from build123d import *

# Parameters (mm, degrees)
BOSS_EXTRUDE1_DEPTH = 5.9944
SKETCH2_R           = 5.08
CUT_EXTRUDE1_DEPTH  = 372.756512027
CUT_EXTRUDE2_DEPTH  = 1.27
FILLET1_R           = 6.35


with BuildPart() as part:
    # Sketch1 → Boss-Extrude1 (new body)
    with BuildSketch(Plane(origin=(0, 0, 0), x_dir=(1, 0, 0), z_dir=(0, 1, 0))):
        Polygon((-66.675, 0), (66.675, 0), (108.238677943, -355.6), (-108.238677943, -355.6), align=None)
    extrude(amount=BOSS_EXTRUDE1_DEPTH)

    # Sketch2 → Cut-Extrude1 (cut, through all)
    with BuildSketch(Plane(origin=(0, 5.9944, 0), x_dir=(1, 0, 0), z_dir=(0, 1, 0))):
        with Locations(Location((0, -101.6, 0), (0, 0, 270))):
            Circle(SKETCH2_R)
    extrude(amount=-CUT_EXTRUDE1_DEPTH, mode=Mode.SUBTRACT)

    # Sketch3 → Cut-Extrude2 (cut)
    with BuildSketch(Plane(origin=(0, 5.9944, 0), x_dir=(1, 0, 0), z_dir=(0, 1, 0))):
        with BuildLine():
            Line((-0.64745098, -125.73), (-7.022352941, -125.73))
            add(Edge.make_bspline(
                [(-7.022352941, -125.73), (-6.995700037, -125.56647139), (-6.94264637, -125.240961184), (-6.822439521, -124.833851847), (-6.660985096, -124.502541973), (-6.475064564, -124.222842773), (-6.235482524, -123.909374898), (-5.933210944, -123.565961589), (-5.569119359, -123.193461978), (-5.137584514, -122.795086731), (-4.639123135, -122.372704423), (-4.278935295, -122.089977316), (-4.090147059, -121.941789216)],
                knots=[0, 0, 0, 0, 1.00794059, 2.006345856, 2.568221262, 3.244176762, 4.045978883, 4.967707078, 6.025786227, 7.214078669, 8.539791974, 10, 10, 10, 10], degree=3))
            add(Edge.make_bspline(
                [(-4.090147059, -121.941789216), (-3.959237505, -121.839291022), (-3.712095896, -121.645786669), (-3.367780634, -121.370812364), (-3.073520037, -121.12638684), (-2.749807849, -120.849934026), (-2.401956914, -120.521669006), (-2.050459284, -120.119964738), (-1.769921232, -119.720001197), (-1.574792785, -119.317093709), (-1.462696622, -118.90576348), (-1.450487068, -118.627391436), (-1.444313725, -118.486642157)],
                knots=[0, 0, 0, 0, 1.105083233, 2.086265203, 2.928643677, 3.647492745, 4.915719202, 6.103603942, 7.190110835, 8.152548768, 9.065899631, 10, 10, 10, 10], degree=3))
            add(Edge.make_bspline(
                [(-1.444313725, -118.486642157), (-1.447965678, -118.383696155), (-1.455062496, -118.183641793), (-1.508208178, -117.89411156), (-1.598896834, -117.626810225), (-1.725875028, -117.381877206), (-1.879897972, -117.157206868), (-2.067602091, -116.959226462), (-2.280144186, -116.783379567), (-2.521172126, -116.634524628), (-2.784585903, -116.511539466), (-3.072628503, -116.429562416), (-3.379272721, -116.373277743), (-3.591834853, -116.369040126), (-3.701053922, -116.366862745)],
                knots=[0, 0, 0, 0, 1.066440105, 2.072406788, 3.038089023, 3.980626898, 4.923164774, 5.851240192, 6.79842777, 7.774055624, 8.779619978, 9.800248095, 10.869719403, 12, 12, 12, 12], degree=3))
            add(Edge.make_bspline(
                [(-3.701053922, -116.366862745), (-3.856272912, -116.372784339), (-4.153856816, -116.384137145), (-4.575842478, -116.488503349), (-4.94872481, -116.662202163), (-5.273158686, -116.90555858), (-5.541086806, -117.223699711), (-5.760536331, -117.605911882), (-5.924737114, -118.058408876), (-5.991270058, -118.385922919), (-6.02627451, -118.558235294)],
                knots=[0, 0, 0, 0, 1.052503955, 2.0178474, 2.928593632, 3.828899676, 4.748107049, 5.732867451, 6.807211463, 8, 8, 8, 8], degree=3))
            Line((-6.02627451, -118.558235294), (-6.823137255, -118.43372549))
            add(Edge.make_bspline(
                [(-6.823137255, -118.43372549), (-6.80933515, -118.324490516), (-6.782336166, -118.110810556), (-6.71294302, -117.80167694), (-6.623223382, -117.510865089), (-6.510230906, -117.238067127), (-6.37723078, -116.983643092), (-6.222961391, -116.746154212), (-6.045126303, -116.528535029), (-5.846128896, -116.329076963), (-5.627309849, -116.151961167), (-5.393797446, -115.994859502), (-5.142464654, -115.86447923), (-4.877381927, -115.754431463), (-4.595667611, -115.670607699), (-4.298686261, -115.611680986), (-3.986147006, -115.577611658), (-3.772730074, -115.57257374), (-3.66370098, -115.57)],
                knots=[0, 0, 0, 0, 1.11558569, 2.182252598, 3.206865404, 4.197163727, 5.171016007, 6.113287932, 7.062752653, 8.014719109, 8.96418383, 9.912249364, 10.862587531, 11.829428462, 12.817713982, 13.836697005, 14.894825442, 16, 16, 16, 16], degree=3))
            add(Edge.make_bspline(
                [(-3.66370098, -115.57), (-3.556720592, -115.572319789), (-3.346239788, -115.576883907), (-3.037889894, -115.614942211), (-2.744018161, -115.6768103), (-2.465296832, -115.763662981), (-2.202890774, -115.877884746), (-1.951202346, -116.010088278), (-1.717482433, -116.17490368), (-1.497639325, -116.359297976), (-1.299748734, -116.564753592), (-1.122645846, -116.782681404), (-0.976555662, -117.018893798), (-0.853169483, -117.266964655), (-0.764695454, -117.53292748), (-0.694872253, -117.809240088), (-0.653577585, -118.101497133), (-0.649522593, -118.30078564), (-0.64745098, -118.402598039)],
                knots=[0, 0, 0, 0, 1.106681904, 2.177364475, 3.209175827, 4.210887483, 5.192078542, 6.167200624, 7.147039734, 8.145062256, 9.132109826, 10.094560107, 11.044836899, 12.000375742, 12.954465884, 13.938765234, 14.946957558, 16, 16, 16, 16], degree=3))
            add(Edge.make_bspline(
                [(-0.64745098, -118.402598039), (-0.651019305, -118.525228757), (-0.6580732, -118.767646194), (-0.715129167, -119.12624646), (-0.813824447, -119.47254261), (-0.943374808, -119.810657932), (-1.113892336, -120.134164725), (-1.314350095, -120.448008584), (-1.547654564, -120.749083332), (-1.770342076, -120.99003171), (-1.97351953, -121.182307301), (-2.148031694, -121.345116208), (-2.346754424, -121.522181935), (-2.570668292, -121.711175794), (-2.818646639, -121.913074715), (-3.084581883, -122.135434202), (-3.377659732, -122.368392422), (-3.582554579, -122.526226013), (-3.688602941, -122.607916667)],
                knots=[0, 0, 0, 0, 1.088993338, 2.152731221, 3.214950677, 4.282992305, 5.363056107, 6.45734114, 7.587448717, 8.741912054, 9.367708333, 10.072059012, 10.861970471, 11.731730561, 12.674646287, 13.702521352, 14.810883478, 16, 16, 16, 16], degree=3))
            add(Edge.make_bspline(
                [(-3.688602941, -122.607916667), (-3.814880187, -122.707673071), (-4.061272368, -122.90231778), (-4.409564614, -123.201952264), (-4.73097902, -123.495186281), (-5.017964452, -123.789920338), (-5.277411759, -124.07905832), (-5.50700849, -124.36473001), (-5.710619134, -124.64507084), (-5.822395863, -124.838757211), (-5.876862745, -124.933137255)],
                knots=[0, 0, 0, 0, 1.201760701, 2.344875646, 3.430713183, 4.449969728, 5.415927222, 6.330865599, 7.186659457, 8, 8, 8, 8], degree=3))
            Line((-5.876862745, -124.933137255), (-0.64745098, -124.933137255))
            Line((-0.64745098, -124.933137255), (-0.64745098, -125.73))
        make_face()
        with BuildLine():
            add(Edge.make_bspline(
                [(7.121960784, -116.348186275), (6.966339865, -116.529937257), (6.658951614, -116.888938584), (6.220934138, -117.43618394), (5.820990618, -117.99084912), (5.449181724, -118.546249507), (5.106128688, -119.103037308), (4.794532343, -119.662337897), (4.516462749, -120.225992354), (4.26698415, -120.792977059), (4.044548147, -121.3683878), (3.850270964, -121.955372575), (3.67057882, -122.552241729), (3.519790538, -123.16358515), (3.387268651, -123.786079212), (3.284032091, -124.423321677), (3.193868357, -125.071600422), (3.156448534, -125.509818618), (3.137647059, -125.73)],
                knots=[0, 0, 0, 0, 1.105388324, 2.183404297, 3.237157451, 4.263515625, 5.270618974, 6.257661546, 7.220201142, 8.173180298, 9.11857031, 10.06900231, 11.029056015, 11.99749775, 12.977109533, 13.9684726, 14.979265319, 16, 16, 16, 16], degree=3))
            Line((3.137647059, -125.73), (2.340784314, -125.73))
            add(Edge.make_bspline(
                [(2.340784314, -125.73), (2.370678975, -125.349642584), (2.429735016, -124.598257492), (2.61102689, -123.492894729), (2.858878127, -122.422284677), (3.182435664, -121.380929429), (3.581330157, -120.3591781), (3.949835575, -119.60787323), (4.230188707, -119.095806913), (4.404577952, -118.809755188), (4.594967573, -118.495142394), (4.815641098, -118.158570547), (5.057471949, -117.794755527), (5.324466786, -117.406124805), (5.619249624, -116.995425039), (5.821900516, -116.712397552), (5.926666667, -116.566078431)],
                knots=[0, 0, 0, 0, 1.601249526, 3.163222193, 4.697516546, 6.211791823, 7.737472103, 9.298034817, 9.721151344, 10.188082837, 10.704348124, 11.265001787, 11.877561367, 12.538519795, 13.244446179, 14, 14, 14, 14], degree=3))
            Line((5.926666667, -116.566078431), (0.94627451, -116.566078431))
            Line((0.94627451, -116.566078431), (0.94627451, -115.769215686))
            Line((0.94627451, -115.769215686), (7.121960784, -115.769215686))
            Line((7.121960784, -115.769215686), (7.121960784, -116.348186275))
        make_face()
    extrude(amount=-CUT_EXTRUDE2_DEPTH, mode=Mode.SUBTRACT)

    # Fillet1
    fillet1_edges = [part.edges().sort_by_distance(p)[0] for p in [
        (108.238677943, 2.9972, 355.6),
        (-108.238677943, 2.9972, 355.6),
        (-66.675, 2.9972, 0),
        (66.675, 2.9972, 0),
    ]]
    fillet(fillet1_edges, radius=FILLET1_R)


solid = part.part
Check sheet for the modelled part. Datum: model origin and axes. Units: mm. Round coordinates to 2 decimals unless told otherwise and drop trailing zeros. Loops run counter-clockwise (first coordinate to the right, second up) from the corner with the lowest first, then second, coordinate; pieces in that order, holes last. Notation, with made-up numbers: (-39.75, -26) -> (-2.75, -26) arc R20 cw to (-2.75, -3) -> close; hole circle Ø9 at (-17, 64.25). An arc over 180 degrees is marked (long way). Put each result on its own line as item: value. Start each with the question number.
1. Section check D-D (z = 247.5). Enter the section's corners in (x, y), plus the area to 3 significant figures.
2. Scan lines: probe 1 along X at (y, z) = (3.2, 101.6); probe 2 along X at (y, z) = (3.15, 136); probe 3 along X at (y, z) = (3.3, 313). Record each from-to range of solid material in increasing order.
3. Section check B-B (y = 1.55). Enter the section's corners in (x, z).
4. Section check C-C (x = -91.5). Enter the section's corners in (y, z), plus the area to 3 significant figures.
5. Draft check along Z on faces 1 (the face through (-87.65, 2.96, 179.46)), 2 (the face through (2, 0, 175)), 3 (the face through (1.526, 3.039, 106.445)). Enter one of: +Z half, -Z half, draft (parallel to the pull), parting line (faces both ways), or undercut.
6. Section check A-A (z = 101.6). Enter the section's corners in (x, y).
7. Gauge pin test, flat ends, axial feed: pin 1 (0.6 mm diameter, centred on y = 5.5, z = 125, fed in from -X); pin 2 (3 mm diameter, centred on y = 3, z = 193.5, fed in from -X); pin 3 (3 mm diameter, centred on y = 1, z = 169, fed in from +X). Record the tip position at first contact, or that the pin passes through.
Findings:
1. outline: (-95.6, 0) -> (95.6, 0) -> (95.6, 5.99) -> (-95.6, 5.99) -> close
1. area: 1,150 mm^2
2. probe 1: x = -78.55 to -5.08, 5.08 to 78.55
2. probe 2: x = -82.57 to 82.57
2. probe 3: x = -103.26 to 103.26
3. outline: (-107.41, 348.51) -> (-67.33, 5.61) arc R6.35 ccw to (-61.02, 0) -> (61.02, 0) arc R6.35 ccw to (67.33, 5.61) -> (107.41, 348.51) arc R6.35 ccw to (101.1, 355.6) -> (-101.1, 355.6) arc R6.35 ccw to start; hole circle Ø10.16 at (0, 101.6)
4. outline: (0, 212.39) -> (5.99, 212.39) -> (5.99, 355.6) -> (0, 355.6) -> close
4. area: 858 mm^2
5. face 1: -Z half
5. face 2: draft
5. face 3: undercut
6. outline: (-78.55, 0) -> (-5.08, 0) -> (-5.08, 5.99) -> (-78.55, 5.99) -> close; (5.08, 0) -> (78.55, 0) -> (78.55, 5.99) -> (5.08, 5.99) -> close
7. pin 1: stops at x = -81.32
7. pin 2: stops at x = -89.47
7. pin 3: stops at x = 86.6
